The figure shows three views and two pictorial views of one solid part (mm, origin at its lowest corner). Answer the questions. A direction names the side the tool comes from. Coordinates: 2 decimals unless noted, no trailing zeros. Order: outer loops, then holes, each group sorted by start corner. A loop starts at its lowest first (then second) coordinate and runs counter-clockwise, first axis right, second up.
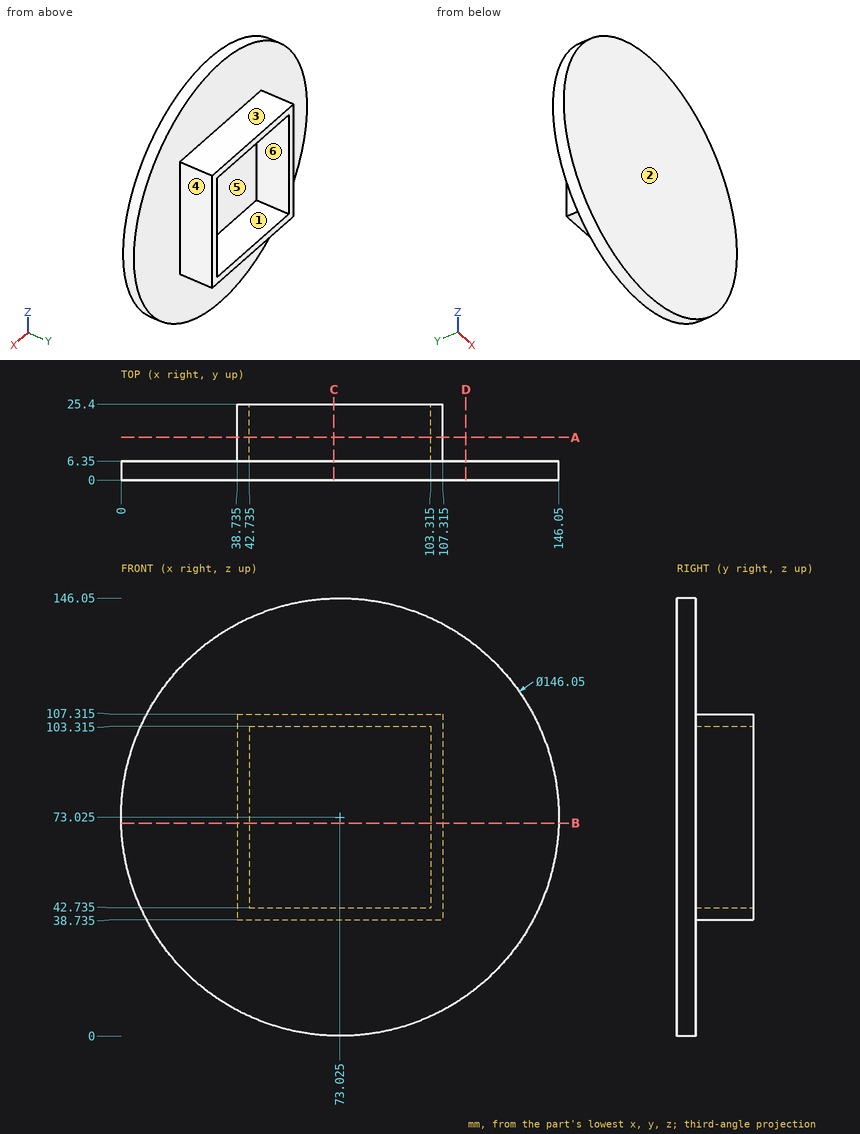
Q1. The part is cut by section C-C, the plane x = 71. Determine the outline of the cut face in (y, z) (3 decimals).
Q2. The part is cut by section B-B, the plane z = 71. Determine the outline of the cut face in (x, y) (3 decimals).
Q3. Straight lines are drawn through the part: L1, parallel to X at y = 24, z = 76 (3 decimals); L2, parallel to Y at x = 118.5, z = 29. For each, find the intervals that lie inside material, in ascending order.
Q4. The part is cut by section D-D, the plane x = 115. Determine the outline of the cut face in (y, z).
Q5. The part is cut by section A-A, the plane y = 14.25. Determine the outline of the cut face in (x, z) (3 decimals).
Q6. Which of the six approach directions +Z, -Z, +X, -X, +Y, -Y give full straight-line access (tool end or side, diameter ignored) to the marked faces 1 and 2?
Q7. Each of these flat-tipped pins is pushed along its axis until it touches: P1, Ø5.5, axis at y = 14.5, z = 84.5, coming from the -X side (3 decimals); P2, Ø10, axis at x = 100, y = 4, coming from the -Z side; P3, Ø12, axis at x = 125.5, z = 89.5, coming from the -Y side; P4, Ø12, axis at y = 3.5, z = 37.5, coming from the +X side. Where does it stop, or does it pass through?
Q8. Determine the mould class of the marked faces 3, 4, 5 and 6 for opening direction Z: +Z half, -Z half, draft (parallel to the pull), parting line (faces both ways), or undercut.
Computed values:
1. outline: (0, 0.028) - (6.35, 0.028) - (6.35, 38.735) - (25.4, 38.735) - (25.4, 42.735) - (6.35, 42.735) - (6.35, 103.315) - (25.4, 103.315) - (25.4, 107.315) - (6.35, 107.315) - (6.35, 146.022) - (0, 146.022) - close
2. outline: (0.028, 0) - (146.022, 0) - (146.022, 6.35) - (107.315, 6.35) - (107.315, 25.4) - (103.315, 25.4) - (103.315, 6.35) - (42.735, 6.35) - (42.735, 25.4) - (38.735, 25.4) - (38.735, 6.35) - (0.028, 6.35) - close
3. L1: x = 38.735 to 42.735, 103.315 to 107.315
3. L2: y = 0 to 6.35
4. outline: (0, 13.27) - (6.35, 13.27) - (6.35, 132.78) - (0, 132.78) - close
5. outline: (38.735, 38.735) - (107.315, 38.735) - (107.315, 107.315) - (38.735, 107.315) - close; hole (42.735, 42.735) - (103.315, 42.735) - (103.315, 103.315) - (42.735, 103.315) - close
6. face 1: +Y
6. face 2: +Z, -Z, +X, -X, -Y
7. P1: stops at x = 38.735
7. P2: stops at z = 3.38
7. P3: stops at y = 0
7. P4: stops at x = 139.82
8. face 3: +Z half
8. face 4: draft
8. face 5: undercut
8. face 6: undercut
